Could you check a few things on this model? Use its own coordinates, in mm. Coordinates: 2 decimals unless noted, no trailing zeros. Loops run counter-clockwise (first coordinate to the right, second up) from the corner with the lowest first, then second, coordinate; pieces in that order, holes last.
1) Imagine slicing it at A-A on x = 0. Please give me the cut outline in (y, z).
2) If I drill on line 1 along Y through (x, z) = (0, 2); line 2 along Y through (x, z) = (-5.5, 1.3), over which ranges is the centre line in solid material (lowest first)?
3) Will this pin go through, and if not, where does the flat tip stop? P1, Ø1.8, axis at x = 0, y = 24.5, coming from the -Z side.
4) Imagine slicing it at B-B on y = 24.5. Please give me the cut outline in (x, z).
5) Imagine slicing it at C-C on z = 2.65. Give the number of separate pieces and of enclosed holes in the cut face, plus the area to 3 significant figures.
```python
from build123d import *

# Parameters (mm, degrees)
SKETCH1_W           = 43
SKETCH1_H           = 74
SKETCH1_R           = 1.5
SKETCH1_W_2         = 5
SKETCH1_H_2         = 5
BOSS_EXTRUDE1_DEPTH = 5


with BuildPart() as part:
    # Sketch1 → Boss-Extrude1 (new body)
    with BuildSketch(Plane.XY):
        with Locations((-5.5, -5)):
            Rectangle(SKETCH1_W, SKETCH1_H)
        Circle(SKETCH1_R, mode=Mode.SUBTRACT)
        with Locations((0, 24.5)):
            Circle(SKETCH1_R, mode=Mode.SUBTRACT)
        with Locations((0, -34.5)):
            Circle(SKETCH1_R, mode=Mode.SUBTRACT)
        with Locations((-7.5, 0)):
            Rectangle(SKETCH1_W_2, SKETCH1_H_2, mode=Mode.SUBTRACT)
        with Locations((7.5, 0)):
            Rectangle(SKETCH1_W_2, SKETCH1_H_2, mode=Mode.SUBTRACT)
        with Locations((-7.5, 24.5)):
            Rectangle(SKETCH1_W_2, SKETCH1_H_2, mode=Mode.SUBTRACT)
        with Locations((7.5, 24.5)):
            Rectangle(SKETCH1_W_2, SKETCH1_H_2, mode=Mode.SUBTRACT)
        with Locations((-7.5, -34.5)):
            Rectangle(SKETCH1_W_2, SKETCH1_H_2, mode=Mode.SUBTRACT)
        with Locations((7.5, -34.5)):
            Rectangle(SKETCH1_W_2, SKETCH1_H_2, mode=Mode.SUBTRACT)
    extrude(amount=BOSS_EXTRUDE1_DEPTH)


solid = part.part
```
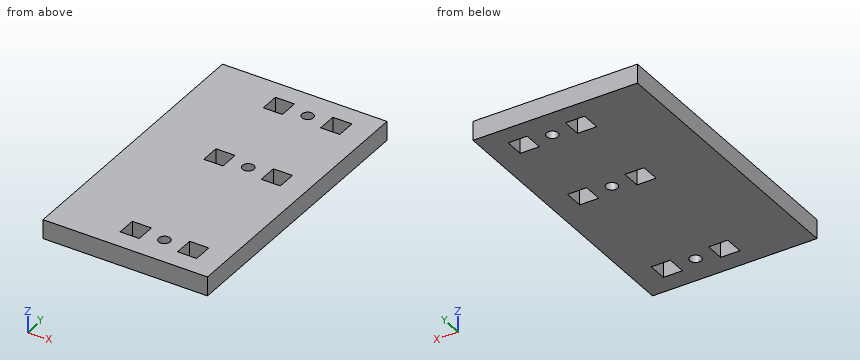
Filled in:
1. outline: (-42, 0) - (-36, 0) - (-36, 5) - (-42, 5) - close; (-33, 0) - (-1.5, 0) - (-1.5, 5) - (-33, 5) - close; (1.5, 0) - (23, 0) - (23, 5) - (1.5, 5) - close; (26, 0) - (32, 0) - (32, 5) - (26, 5) - close
2. line 1: y = -42 to -36, -33 to -1.5, 1.5 to 23, 26 to 32
2. line 2: y = -42 to -37, -32 to -2.5, 2.5 to 22, 27 to 32
3. P1: passes through
4. outline: (-27, 0) - (-10, 0) - (-10, 5) - (-27, 5) - close; (-5, 0) - (-1.5, 0) - (-1.5, 5) - (-5, 5) - close; (1.5, 0) - (5, 0) - (5, 5) - (1.5, 5) - close; (10, 0) - (16, 0) - (16, 5) - (10, 5) - close
5. separate pieces: 1
5. enclosed holes: 9
5. area: 3,010 mm2
